Autodesk Inventor part; units mm, degrees
ref_plane "YZ Plane" through (0, 0, 0) normal (1, 0, 0) x (0, 1, 0)
ref_plane "XZ Plane" through (0, 0, 0) normal (0, 1, 0) x (-1, 0, 0)
ref_plane "XY Plane" through (0, 0, 0) normal (0, 0, 1) x (1, 0, 0)
sketch "Эскиз1" plane through (0, 0, 0) normal (0, 0, 1) x (1, 0, 0)
  spline S0 degree 3 number of poles 571 construction
  circle A0 centre (0, 0) radius 12.4728
  circle A1 centre (0, 0) radius 11.6873
  spline S1 degree 3 number of poles 571 construction
  circle A2 centre (0.0593, 50) radius 3.05 construction
  circle A3 centre (0.0593, 50) radius 12.4622
  circle A4 centre (0.0593, 50) radius 11.6915
  line L0 (12.5215, 49.9878) -> (12.4728, -0.0121)
  line L1 (-12.4028, 50.0174) -> (-12.4728, 0.0175)
  line L2 (-11.6322, 50.0129) -> (-11.6873, 0.0129)
  line L3 (-11.6921, -4.3435) -> (-11.689, -1.4984)
  line L4 (11.7508, 49.9851) -> (11.6873, -0.0148)
  line L5 (0, 0) -> (-30.3964, 0.0335) construction
  point P0 (-23.5791, 58.2576)
  point P1 (2.2116, 51.4848)
  point P2 (12.4728, 0)
  dimension "d0" = 24.9244
  dimension "d1" = 24.9457
  dimension "d2" = 23.383
  dimension "d3" = 23.3746
  dimension "d6" = 50
extrude "Выдавливание1" add sketch "Эскиз1" along normal blind 6 contours A0 L2 A1 L4 | L1 A3 L2 A0 | A3 L4 A4 L2 | L4 A3 L0 A0 picked at (-11.8082, -1.4117) picked at (12.144, 50.9937)
properties part number "Ремень"
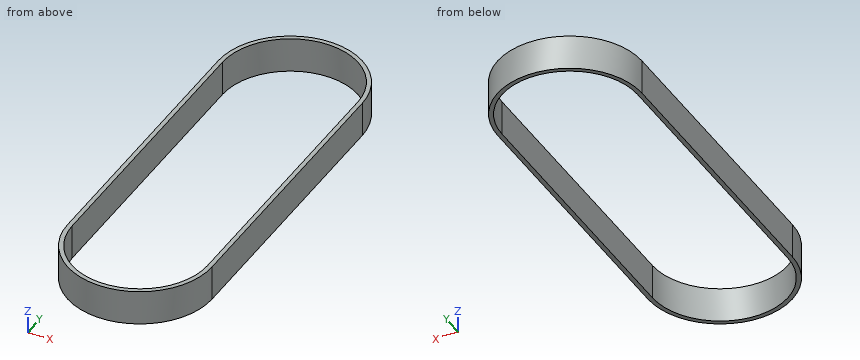
Geometry check sheet. Reference: the model listing, model coordinates, mm. Coordinates: 2 decimals unless noted, no trailing zeros. Loops run counter-clockwise (first coordinate to the right, second up) from the corner with the lowest first, then second, coordinate; pieces in that order, holes last. Notation, with made-up numbers: (37.25, 21) - (88.25, 21) arc R3 cw to (88.25, 25) - close; hole circle Ø9 at (89.25, 41.5). An arc over 180 degrees is marked (long way). Use one line per item in the form item = value. Start each with the question number.
Item 1: Section check A-A, the plane y = 45. Enter the section's corners in (x, z), and give its area (3 significant figures).
Item 2: Thickness scan on probe 1 along X at (y, z) = (11, 3.25); probe 2 along X at (y, z) = (49, 1.8); probe 3 along Y at (x, z) = (7.5, 1.2). Record the ranges inside material, lowest first.
Item 3: Section check B-B, the plane x = 4. Enter the section's corners in (y, z), and give its area (3 significant figures).
Item 4: Gauge pin test, flat end, axial feed: pin 1 (2 mm diameter, centred on y = 51, z = 4.5, fed in from -X). Record the tip position at first contact, or that the pin passes through.
Item 5: Section check C-C, the plane z = 1.9. Enter the section's corners in (x, y).
Computed:
q1.outline = (-12.41, 0) - (-11.64, 0) - (-11.64, 6) - (-12.41, 6) - close; (11.74, 0) - (12.52, 0) - (12.52, 6) - (11.74, 6) - close
q1.area = 9.27 mm2
q2.probe_1 = -12.46 to -11.68, 11.7 to 12.48
q2.probe_2 = -12.4 to -11.63, 11.75 to 12.52
q2.probe_3 = -9.97 to -8.96, 59.02 to 60
q3.outline = (-11.81, 0) - (-10.98, 0) - (-10.98, 6) - (-11.81, 6) - close; (61.01, 0) - (61.82, 0) - (61.82, 6) - (61.01, 6) - close
q3.area = 9.89 mm2
q4.pin_1 = -12.4
q5.outline = (-12.47, 0.02) arc R12.47 ccw to (12.47, 0) - (12.52, 49.99) arc R12.46 ccw to (-12.4, 50.02) - close; hole (-11.69, 0.01) arc R11.69 ccw to (11.69, 0) - (11.75, 49.99) arc R11.69 ccw to (-11.63, 50.01) - close
